```python
from build123d import *

# Parameters (mm, degrees)
F1_DEPTH     = 55
F1_TAPER     = -15
F4_DEPTH     = 55
F4_TAPER     = -12
F5_W         = 5
F5_H         = 130
F6_DEPTH     = 47
F10_W        = 360.01701653
F10_H        = 225.87454319
F11_DEPTH    = 25
F12_W        = 5
F12_H        = 46
F13_DEPTH    = 10
F14_W        = 5
F14_H        = 46
F15_DEPTH    = 10
F8_W         = 54.0339685977
F8_H         = 90.1
F16_DEPTH    = 32.6
F9_W         = 55.9400806222
F9_H         = 89.7377200425
F17_DEPTH    = 25
F18_W        = 347.7291613817
F18_H        = 217.2330617905
F19_DEPTH    = 25
F20_W        = 34.4053636551
F20_H        = 45.9854951713
F21_DEPTH    = 25
F22_W        = 1.5565819549
F22_H        = 85.7377200425
F22_W_2      = 27.4434180451
F23_DEPTH    = 52
F24_T1_DEPTH = 114.7377200425


# Not quite as in the source:
# - a fillet or chamfer that OpenCascade refuses, or shapes differently, is made with other operations: its cross-section is extruded or revolved along the edge and cut away or added


with BuildPart() as f1:
    # F0 (on Front) → F1 (new body)
    with BuildSketch(Plane.XZ):
        with BuildLine():
            Line((34.0782237053, 85.1892769337), (-105.9217762947, 85.1892769337))
            ThreePointArc((-105.9217762947, 85.1892769337), (-120.0639119184, 79.3314125574), (-125.9217762947, 65.1892769337))
            Line((-125.9217762947, 65.1892769337), (-125.9217762947, -24.8107230663))
            ThreePointArc((-125.9217762947, -24.8107230663), (-120.0639119184, -38.9528586901), (-105.9217762947, -44.8107230663))
            Line((-105.9217762947, -44.8107230663), (34.0782237053, -44.8107230663))
            ThreePointArc((34.0782237053, -44.8107230663), (48.220359329, -38.9528586901), (54.0782237053, -24.8107230663))
            Line((54.0782237053, -24.8107230663), (54.0782237053, 65.1892769337))
            ThreePointArc((54.0782237053, 65.1892769337), (48.220359329, 79.3314125574), (34.0782237053, 85.1892769337))
        make_face()
    extrude(amount=F1_DEPTH, taper=F1_TAPER)

    # F3 (on offset) → F4 (cut)
    with BuildSketch(Plane.XZ.offset(5)):
        with BuildLine():
            Line((34.106137666, 85.2195297501), (-105.893862334, 85.2195297501))
            ThreePointArc((-105.893862334, 85.2195297501), (-120.0359979577, 79.3616653739), (-125.893862334, 65.2195297501))
            Line((-125.893862334, 65.2195297501), (-125.893862334, -24.7804702499))
            ThreePointArc((-125.893862334, -24.7804702499), (-120.0359979577, -38.9226058736), (-105.893862334, -44.7804702499))
            Line((-105.893862334, -44.7804702499), (34.106137666, -44.7804702499))
            ThreePointArc((34.106137666, -44.7804702499), (48.2482732898, -38.9226058736), (54.106137666, -24.7804702499))
            Line((54.106137666, -24.7804702499), (54.106137666, 65.2195297501))
            ThreePointArc((54.106137666, 65.2195297501), (48.2482732898, 79.3616653739), (34.106137666, 85.2195297501))
        make_face()
    extrude(amount=F4_DEPTH, taper=F4_TAPER, mode=Mode.SUBTRACT)

    # F5 (on face) → F6 (join)
    with BuildSketch(Plane.XZ.offset(5)):
        with Locations((-35.893862334, 20.2195297501)):
            Rectangle(F5_W, F5_H)
    extrude(amount=F6_DEPTH)

    # F10 (on Front) → F11 (cut)
    with BuildSketch(Plane.XZ):
        with Locations((5.3876563907, 10.9746605158)):
            Rectangle(F10_W, F10_H)
    extrude(amount=-F11_DEPTH, mode=Mode.SUBTRACT)

    # F12 (on face) → F13 (join)
    with BuildSketch(Plane(origin=(0, 8.8907927165, -41.8278911112), x_dir=(1, 0, 0), z_dir=(0, -0.2079116908, 0.9781476007))):
        with Locations((-35.893862334, -37.2011212889)):
            Rectangle(F12_W, F12_H)
    extrude(amount=F13_DEPTH)

    # F14 (on face) → F15 (join)
    with BuildSketch(Plane(origin=(0, 17.1148163716, 80.5188804202), x_dir=(1, 0, 0), z_dir=(0, -0.2079116908, -0.9781476007))):
        with Locations((-35.893862334, 45.6088745247)):
            Rectangle(F14_W, F14_H)
    extrude(amount=F15_DEPTH)

    # F8 (on offset) → F16 (join)
    with BuildSketch(Plane.YZ.offset(98)):
        with Locations((-27.0169842988, 19.8769969761)):
            Rectangle(F8_W, F8_H)
    extrude(amount=-F16_DEPTH)

    # F9 (on face) → F17 (join)
    with BuildSketch(Plane(origin=(50.4556696128, 13.5195559263, 0), x_dir=(-0.2588190451, 0.9659258263, 0), z_dir=(0.9659258263, 0.2588190451, 0))):
        with Locations((-41.9665145313, 20.0581369549)):
            Rectangle(F9_W, F9_H)
    extrude(amount=F17_DEPTH)

    # F18 (on Front) → F19 (cut)
    with BuildSketch(Plane.XZ):
        with Locations((0.111065805, 20.1892703772)):
            Rectangle(F18_W, F18_H)
    extrude(amount=-F19_DEPTH, mode=Mode.SUBTRACT)

    # F20 (on face) → F21 (cut)
    with BuildSketch(Plane(origin=(0, 0, -24.8107230663), x_dir=(1, 0, 0), z_dir=(0, 0, -1))):
        Polygon((68.0166854944, 55.7510983837), (65.4, 45.9854951713), (99.8053636551, 45.9854951713), (100.283839941, 55.7510983837), align=None)
        with Locations((82.6026818275, 22.9927475857)):
            Rectangle(F20_W, F20_H)
    extrude(amount=F21_DEPTH, mode=Mode.SUBTRACT)

    # F22 (on face) → F23 (cut)
    with BuildSketch(Plane.XZ.offset(54.0339685977)):
        with Locations((67.7782909774, 20.0581369549)):
            Rectangle(F22_W, F22_H)
        with Locations((82.2782909774, 20.0581369549)):
            Rectangle(F22_W_2, F22_H)
    extrude(amount=-F23_DEPTH, mode=Mode.SUBTRACT)

    # F24: fillet of radius 5 on 2 edges, made by hand

    # F24_s2 → F24_t1 (cut)
    with BuildSketch(Plane.XY.offset(-37.3107230663)):
        with BuildLine():
            ThreePointArc((98, -49.0339685977), (96.5355339059, -52.5695025036), (93, -54.0339685977))
            Line((93, -54.0339685977), (98, -54.0339685977))
            Line((98, -54.0339685977), (98, -49.0339685977))
        make_face()
        with BuildLine():
            ThreePointArc((93, 0), (96.5355339059, -1.4644660941), (98, -5))
            Line((98, -5), (98, 0))
            Line((98, 0), (93, 0))
        make_face()
    extrude(amount=F24_T1_DEPTH, mode=Mode.SUBTRACT)


solid = f1.part
```
Verification items for the finished model (mm, model axes). A direction names the side the tool comes from. Coordinates: 2 decimals unless noted, no trailing zeros. Return JSON: item names as keys, results as strings.
(1) Access from +Z, -Z, +X, -X, +Y, -Y to the whole of each face (thin tool, end or side, straight path). Record for faces 1 (the flat face through (-35.93, -51.02, -49.52)), 2 (the cylindrical face through (97.554, -51.097, 19.43)), 3 (the flat face through (81, -28, -24.811)).
Filled sheet:
{"face 1": "-Y", "face 2": "+Z, -Z, +X, -Y", "face 3": "-Z, +X, +Y"}
(2) Section check A-A, the plane y = -23.5. Give the number of separate pieces and of enclosed holes in the cut face, and give its area (3 significant figures).
Filled sheet:
{"separate pieces": "1", "enclosed holes": "3", "area": "3,040 mm^2"}
(3) Mould release check, pull along X, two halves, no side actions. Record for faces 4 (the flat face through (98, -27, 21)), 5 (the flat face through (-36, -52, 21)), 6 (the conical face through (-125.56, -27.88, -44.02)), 7 (the flat face through (-60, -55, -57)): pulls with the +X half, pulls with the -X half, needs draft (parallel to the pull), parting line crosses it, or undercut.
Filled sheet:
{"face 4": "pulls with the +X half", "face 5": "undercut", "face 6": "pulls with the -X half", "face 7": "needs draft"}
(4) Go/stop test with flat-tipped pins: pin 1 (1.5 mm diameter, centred on y = -37, z = -33.5, fed in from +X); pin 2 (22 mm diameter, centred on x = 66.5, y = -18, fed in from -Z); pin 3 (23.5 mm diameter, centred on y = -34.5, z = -14.5, fed in from -X). Record where each tip stops, or that it passes through.
Filled sheet:
{"pin 1": "stops at x = 63.01", "pin 2": "stops at z = -38.23", "pin 3": "stops at x = -138.31"}
(5) Thickness scan on line 1 along X through (y, z) = (-44.5, 54.5); line 2 along X through (y, z) = (-21, 60); line 3 along X through (y, z) = (-6, 82.5). Record the ranges inside material, lowest first.
Filled sheet:
{"line 1": "x = -137.85 to -134.29, -38.39 to -33.39, 62.5 to 67, 96 to 98", "line 2": "x = -131.55 to -129.29, -38.39 to -33.39, 57.51 to 67, 96 to 98", "line 3": "x = -118.85 to -116.38, -38.39 to -33.39, 44.59 to 47.01"}
